Autodesk Inventor part; units mm, degrees
ref_plane "YZ Plane" through (0, 0, 0) normal (1, 0, 0) x (0, 1, 0)
ref_plane "XZ Plane" through (0, 0, 0) normal (0, 1, 0) x (-1, 0, 0)
ref_plane "XY Plane" through (0, 0, 0) normal (0, 0, 1) x (1, 0, 0)
sketch "Sketch5" plane through (0, 0, 0) normal (0, 1, 0) x (-1, 0, 0)
  line L0 (-22.5, 13) -> (22.5, 13) construction
  line L1 (8, 13) -> (8, 0)
  line L2 (8, 0) -> (34.925, 0)
  line L3 (34.925, 0) -> (34.925, 13)
  line L4 (34.925, 13) -> (11.9, 13)
  line L5 (11.9, 11.8) -> (9.5, 11.8)
  line L6 (9.5, 11.8) -> (9.5, 13)
  line L7 (11.9, 11.8) -> (11.9, 13)
  line L8 (0, -1.501) -> (0, 14.3549) construction
  line L9 (8, 13) -> (9.5, 13)
  dimension "d38" = 13
  dimension "d39" = 8
  dimension "d40" = 9.5
  dimension "d41" = 2.4
  dimension "d42" = 1.2
  dimension "d43" = 34.925
ref_plane "Work Plane1" through (0, 0, 13) normal (0, 0, -1) x (-1, 0, 0)
revolve "Revolution1" add sketch "Sketch5" angle 360 about axis through (0, 0, -1.501) along (0, 0, 1)
sketch "Sketch9" plane through (0, 0, 13) normal (0, 0, 1) x (1, 0, 0)
  circle A0 centre (0, 0) radius 11.9
  circle A1 centre (0, 0) radius 17.5
  circle A2 centre (0, 0) radius 17.5
  circle A3 centre (0, 0) radius 17.5
  circle A4 centre (0, 0) radius 17.5
  circle A5 centre (0, 0) radius 17.5
  circle A6 centre (0, 0) radius 17.5
  point P0 (0, 17.5)
  point P1 (-15.1554, 8.75)
  point P2 (-15.1554, -8.75)
  point P3 (0, -17.5)
  point P4 (15.1554, -8.75)
  point P5 (15.1554, 8.75)
  dimension "d75" = 35
  dimension "d78" = 360
hole "Hole6" at (0, 17.5, 13) at (-15.1554, 8.75, 13) at (-15.1554, -8.75, 13) at (0, -17.5, 13) at (15.1554, -8.75, 13) at (15.1554, 8.75, 13) direction (0, 0, -1) diameter 3.242 depth 7 tip angle 118
sketch "Sketch10" plane through (0, 0, 13) normal (0, 0, 1) x (1, 0, 0)
  circle A0 centre (0, 0) radius 11.9
  circle A1 centre (0, 0) radius 29.35
  point P0 (0, 29.35)
  point P1 (-25.4178, 14.675)
  point P2 (-25.4178, -14.675)
  point P3 (0, -29.35)
  point P4 (25.4178, -14.675)
  point P5 (25.4178, 14.675)
  dimension "d87" = 58.7
  dimension "d90" = 360
hole "Hole7" at (0, 29.35, 13) at (-25.4178, 14.675, 13) at (-25.4178, -14.675, 13) at (0, -29.35, 13) at (25.4178, -14.675, 13) at (25.4178, 14.675, 13) direction (0, 0, -1) diameter 6.7 end through all
properties part number "Conflat Flange"
Build history of the part. All positions in model axes, mm. A direction names the side the tool comes from. Round coordinates to 2 decimals unless told otherwise and drop trailing zeros. Write each loop counter-clockwise with the first axis right and the second up, starting at its lowest first coordinate (ties: lowest second). Pieces come first, ordered by that corner, then holes. Notation, with made-up numbers: M -31.75,32 L -10.75,32 A27 ccw -10.75,50 Z; hole C 70,68 d3. An arc over 180 degrees is marked long. Answer as a JSON object with one key per item and string values. Group by question number.
(1) Which spindle directions (+Z, -Z, +X, -X, +Y, -Y) get a long thin tool onto all of the face, cutting with end or side? Do faces 5 (the cylindrical face through (-0.487, 15.954, 9.451)), 6 (the cylindrical face through (-1.006, 26.155, 6.409)). Say none if no direction does.
(2) Mould opens along Y. For faces 1 (the cylindrical face through (27.715, 21.251, 6.591)), 2 (the flat face through (0, 15, 13)), 3 (the cylindrical face through (-25.57, -11.33, 6.41)), 4 (the flat face through (1, 10, 11.8)) say: pulls with the +Y half, pulls with the -Y half, needs draft (parallel to the pull), parting line crosses it, or undercut.
(3) Cut at B-B (x = 6). Give the cut face in (y, z).
(4) Cut at A-A (y = 0). Give the cut face in (x, z) (3 decimals).
(5) Flat gauge pins, fed straight in: pin 1 (1 mm diameter, centred on x = -20, z = 11.5, fed in from -Y); pin 2 (5.5 mm diameter, centred on x = -25.42, y = -14.68, fed in from -Z); pin 3 (4 mm diameter, centred on y = -17, z = 4, fed in from -X); pin 4 (1.9 mm diameter, centred on x = 0, y = -17.5, fed in from +Z). Where does each tip first touch, or does it go through?
(6) Drill centre lines: L1, parallel to Y at x = 0, z = 4.75 (3 decimals); L2, parallel to X at y = -17, z = 10.5; L3, parallel to Y at x = 15.5, z = 7.75. Where is each one in solid material? Low to high.
(7) Cut at C-C (z = 3.75). Give the cut face in (x, y) (3 decimals), and give its area (3 significant figures).
(8) Cut at D-D (y = 13). Give the cut face in (x, z), and give its area (3 significant figures).
Responses:
{
 "1": {"face 5": "+Z", "face 6": "+Z, -Z"},
 "2": {"face 1": "parting line crosses it", "face 2": "needs draft", "face 3": "undercut", "face 4": "undercut"},
 "3": {"outline": "M -34.41,0 L -5.29,0 L -5.29,13 L -7.37,13 L -7.37,11.8 L -10.28,11.8 L -10.28,13 L -34.41,13 Z; M 5.29,0 L 34.41,0 L 34.41,13 L 10.28,13 L 10.28,11.8 L 7.37,11.8 L 7.37,13 L 5.29,13 Z"},
 "4": {"outline": "M -34.925,0 L -8,0 L -8,13 L -9.5,13 L -9.5,11.8 L -11.9,11.8 L -11.9,13 L -34.925,13 Z; M 8,0 L 34.925,0 L 34.925,13 L 11.9,13 L 11.9,11.8 L 9.5,11.8 L 9.5,13 L 8,13 Z"},
 "5": {"pin 1": "stops at y = -28.97", "pin 2": "passes through", "pin 3": "stops at x = -31.54", "pin 4": "stops at z = 5.6"},
 "6": {"L1": "y = -34.925 to -32.7, -26 to -8, 8 to 26, 32.7 to 34.925", "L2": "x = -30.51 to -27.83, -23.01 to -1.54, 1.54 to 23.01, 27.83 to 30.51", "L3": "y = -31.3 to -10.33, -7.17 to 7.17, 10.33 to 31.3"},
 "7": {"outline": "C 0,0 d69.85; hole C -25.418,-14.675 d6.7; hole C -25.418,14.675 d6.7; hole C 0,0 d16; hole C 0,-29.35 d6.7; hole C 0,29.35 d6.7; hole C 25.418,-14.675 d6.7; hole C 25.418,14.675 d6.7", "area": "3,420 mm2"},
 "8": {"outline": "M -32.42,0 L -28.32,0 L -28.32,13 L -32.42,13 Z; M -22.52,0 L 22.52,0 L 22.52,13 L -22.52,13 Z; M 28.32,0 L 32.42,0 L 32.42,13 L 28.32,13 Z", "area": "692 mm2"}
}
